Geometry check sheet. Reference: the model listing, model coordinates, mm. A direction names the side the tool comes from. Give positions to 0.01 mm unless a question says otherwise; leave off trailing zeros. Order: outer loops, then holes, each group sorted by start corner. A loop starts at its lowest first (then second) coordinate and runs counter-clockwise, first axis right, second up. Notation, with made-up numbers: M 22,55 L 32,55 A24 cw 32,83 Z; hole C 45.25,89.25 d10. An arc over 180 degrees is marked long. Answer as a JSON object with one key per item and string values. Group by question number.
from build123d import *

# Parameters (mm, degrees)
SKETCH1_W           = 250
SKETCH1_H           = 250
BOSS_EXTRUDE1_DEPTH = 20
SKETCH2_R           = 100
BOSS_EXTRUDE2_DEPTH = 100
SKETCH3_R           = 70
BOSS_EXTRUDE3_DEPTH = 100
SKETCH4_R           = 100
BOSS_EXTRUDE4_DEPTH = 10


with BuildPart() as part:
    # Sketch1 → Boss-Extrude1 (new body)
    with BuildSketch(Plane(origin=(0, 0, 0), x_dir=(1, 0, 0), z_dir=(0, 1, 0))):
        with Locations((46.810699588, -38.16872428)):
            Rectangle(SKETCH1_W, SKETCH1_H)
    extrude(amount=BOSS_EXTRUDE1_DEPTH)

    # Sketch2 → Boss-Extrude2 (add)
    with BuildSketch(Plane(origin=(0, 20, 0), x_dir=(1, 0, 0), z_dir=(0, 1, 0))):
        with Locations(Location((46.810699588, -38.16872428, 0), (0, 0, 270))):
            Circle(SKETCH2_R)
    extrude(amount=BOSS_EXTRUDE2_DEPTH)

    # Sketch3 → Boss-Extrude3 (add)
    with BuildSketch(Plane(origin=(0, 120, 0), x_dir=(1, 0, 0), z_dir=(0, 1, 0))):
        with Locations(Location((46.810699588, -38.16872428, 0), (0, 0, 270))):
            Circle(SKETCH3_R)
    extrude(amount=BOSS_EXTRUDE3_DEPTH)

    # Sketch4 → Boss-Extrude4 (add)
    with BuildSketch(Plane(origin=(0, 220, 0), x_dir=(1, 0, 0), z_dir=(0, 1, 0))):
        with Locations(Location((46.810699588, -38.16872428, 0), (0, 0, 270))):
            Circle(SKETCH4_R)
    extrude(amount=BOSS_EXTRUDE4_DEPTH)


solid = part.part
1. Depth check by flat-ended pin: pin 1 (2 mm diameter, centred on y = 60.5, z = 1.5, fed in from -X); pin 2 (5 mm diameter, centred on y = 130.5, z = -28, fed in from +X); pin 3 (12 mm diameter, centred on x = 114, y = 165.5, fed in from -Z). Enter the tip coordinate at first touch or a pass-through.
2. Thickness scan on line 1 along Y through (x, z) = (128, 46.5); line 2 along Y through (x, z) = (-55, 103); line 3 along X through (y, z) = (68.5, -32). Record the ranges inside material, lowest first. Write a range as [from, to].
3. Cross-section at B-B (z = 35.5). Record the cut outline in (x, y), and give its area (3 significant figures).
4. Release check for a two-part mould opening along Y. For faces 4 (the flat face through (26, 220, -30)), 5 (the flat face through (45, 10, 163.169)), 6 (the flat face through (45, 0, 36)) record: released by +Y, released by -Y, zero draft, split by the parting line, or undercut.
5. Cross-section at A-A (x = 123). Record the cut outline in (y, z), and give its area (3 significant figures).
6. Cross-section at D-D (y = 148). Record the cut outline in (x, z), and give its area (3 significant figures).
7. Access from +Z, -Z, +X, -X, +Y, -Y to the whole of each face (thin tool, end or side, straight path). Record for faces 1 (the flat face through (48, 230, 37)), 2 (the cylindrical face through (105.835, 169.3, 75.8)), 3 (the flat face through (-10, 20, -47)).
8. Cross-section at C-C (x = 54). Record the cut outline in (y, z), and give its area (3 significant figures).
Report:
{
 "1": {"pin 1": "stops at x = -46.61", "pin 2": "stops at x = 75.9", "pin 3": "stops at z = 4.17"},
 "2": {"line 1": "y = [0, 120], [220, 230]", "line 2": "y = [0, 20]", "line 3": "x = [-24.44, 118.06]"},
 "3": {"outline": "M -78.19,0 L 171.81,0 L 171.81,20 L 146.78,20 L 146.78,120 L 116.76,120 L 116.76,220 L 146.78,220 L 146.78,230 L -53.15,230 L -53.15,220 L -23.14,220 L -23.14,120 L -53.15,120 L -53.15,20 L -78.19,20 Z", "area": "41,000 mm2"},
 "4": {"face 4": "undercut", "face 5": "zero draft", "face 6": "released by -Y"},
 "5": {"outline": "M 0,-86.83 L 20,-86.83 L 20,-26.6 L 120,-26.6 L 120,102.94 L 20,102.94 L 20,163.17 L 0,163.17 Z; M 220,-26.6 L 230,-26.6 L 230,102.94 L 220,102.94 Z", "area": "19,200 mm2"},
 "6": {"outline": "C 46.81,38.17 d140", "area": "15,400 mm2"},
 "7": {"face 1": "+Z, -Z, +X, -X, +Y", "face 2": "none", "face 3": "+Y"},
 "8": {"outline": "M 0,-86.83 L 20,-86.83 L 20,-61.57 L 120,-61.57 L 120,-31.46 L 220,-31.46 L 220,-61.57 L 230,-61.57 L 230,137.91 L 220,137.91 L 220,107.8 L 120,107.8 L 120,137.91 L 20,137.91 L 20,163.17 L 0,163.17 Z", "area": "40,900 mm2"}
}
